Autodesk Fusion 360 part; units mm, degrees
sketch "Esquisse1" plane through (0, 0, 0) normal (0, 0, 1) x (1, 0, 0)
  circle A0 centre (0, 0) radius 6.5
  circle A1 centre (0, 64) radius 6.5
  line L0 (0, 64) -> (0, 0)
  line L1 (0, 64) -> (-6.5, 64)
  line L2 (0, 64) -> (6.5, 64)
  line L3 (0, 0) -> (6.5, 0)
  line L4 (0, 0) -> (-6.5, 0)
  line L5 (-6.5, 64) -> (-6.5, 0)
  line L6 (6.5, 64) -> (6.5, 0)
  line L7 (0, 64) -> (0, 44.5)
  line L8 (-2.75, 47.25) -> (2.75, 47.25)
  circle A2 centre (0, 47.25) radius 2.75
  line L9 (-2.75, 47.25) -> (-6.3285, 62.5166)
  line L10 (2.75, 47.25) -> (6.3285, 62.5166)
  dimension "d1" = 13
  dimension "d2" = 13
  dimension "d3" = 64
  dimension "d4" = 19.5
  dimension "d5" = 5.5
  dimension "d6" = 2.75
  dimension "d7" = 2.75
extrude "Extrusion1" add sketch "Esquisse1" along normal blind 3
extrude "Extrusion2" add sketch "Esquisse1" against normal blind 2 contours A0 L3 L4 | A0 A1 L0 L5 A2 L9 | A0 L0 L4 | A0 L0 L3 | A0 A1 L0 L6 A2 L10
sketch "Esquisse2" plane through (0, 0, 3) normal (0, 0, 1) x (-1, 0, 0)
  line L0 (6.5, -64) -> (6.5, 0)
  arc A0 (6.5, 0) -> (-6.5, 0) centre (0, 0) ccw
  line L1 (-6.5, 0) -> (-6.5, -64)
  arc A1 (-6.5, -64) -> (6.5, -64) centre (0, -64) ccw
  circle A2 centre (0, 0) radius 1.5
  circle A3 centre (0, -64) radius 1.5
  dimension "d12" = 3
  dimension "d13" = 3
extrude "Extrusion3" cut sketch "Esquisse2" against normal blind 5 contours A2 | A3
sketch "Esquisse3" plane through (0, 0, 3) normal (0, 0, 1) x (-1, 0, 0)
  circle A0 centre (0, -64) radius 1.5
  circle A1 centre (0, 0) radius 1.5
  line L0 (6.5, -64) -> (6.5, 0)
  arc A2 (6.5, 0) -> (-6.5, 0) centre (0, 0) ccw
  line L1 (-6.5, 0) -> (-6.5, -64)
  arc A3 (-6.5, -64) -> (6.5, -64) centre (0, -64) ccw
  circle A4 centre (0, -64) radius 1.5
  circle A5 centre (0, -64) radius 3.5
  circle A6 centre (0, 0) radius 1.5
  circle A7 centre (0, 0) radius 3.5
  dimension "d16" = 7
  dimension "d17" = 3
  dimension "d18" = 3
  dimension "d19" = 7
extrude "Extrusion5" add sketch "Esquisse3" along normal blind 2 contours A5 | A7
Source: CAD feature listing. Evaluate the final solid. Frame: model axes, mm. A direction names the side the tool comes from. Coordinates: 2 decimals unless noted, no trailing zeros. Loops run counter-clockwise (first coordinate to the right, second up) from the corner with the lowest first, then second, coordinate; pieces in that order, holes last. Notation, with made-up numbers: M 41.5,-32.5 L 85.5,-32.5 A21 ccw 85.5,-5.5 Z; hole C 29.5,60.5 d5. An arc over 180 degrees is marked long. Use a Markdown table: item, result. Add a question column.
Q1. First-contact query: pin 1 (4 mm diameter, centred on x = 3, z = -0.5, fed in from +Y); pin 2 (1.5 mm diameter, centred on x = 4.5, z = 4, fed in from +Y); pin 3 (4 mm diameter, centred on x = -0.5, y = 57.5, fed in from -Z); pin 4 (1.5 mm diameter, centred on x = -4, y = 56.5, fed in from +Z). Flat tips, straight axial feed; report the tip coordinate or a pass-through.
Q2. Material intervals for L1, parallel to Y at x = 0, z = 1.1; L2, parallel to X at y = 64, z = 1.65; L3, parallel to Y at x = 0, z = 3.2, sorted ascending.
Q3. Section query B-B, the plane z = 2.25. Return loops of the section in (x, y), and give its area (3 significant figures).
Q4. Access query for faces 1 (the cylindrical face through (0.1, -6.5, 0.5)), 2 (the flat face through (0, 58, 0)), 3 (the cylindrical face through (-3.233, -1.341, 3.986)). Directions: +Z, -Z, +X, -X, +Y, -Y. A direction counts if a zero-diameter tool reaches every point of the face in a straight line with its end or side. Return the directions, or none.
Q5. Draft query along X for faces 4 (the cylindrical face through (-0.806, 65.265, 2.465)), 5 (the cylindrical face through (1.5, 0.07, 1.45)), 6 (the flat face through (0, 66, 5)), 7 (the cylindrical face through (-1.88, 66.95, 3.99)). Return one class per face: pulls with the +X half, pulls with the -X half, needs draft (parallel to the pull), parting line crosses it, or undercut.
Q6. Section query A-A, the plane x = 0. Return loops of the section in (y, z), and give its area (3 significant figures).
Q7. Section query D-D, the plane x = 4.75. Return loops of the section in (y, z), and give its area (3 significant figures).
Q8. Section query C-C, the plane z = -1.25. Return loops of the section in (x, y).
Result:
| question | item | result |
|---|---|---|
| 1 | pin 1 | stops at y = 70.41 |
| 1 | pin 2 | passes through |
| 1 | pin 3 | stops at z = 0 |
| 1 | pin 4 | stops at z = 3 |
| 2 | L1 | y = -6.5 to -1.5, 1.5 to 62.5, 65.5 to 70.5 |
| 2 | L2 | x = -6.5 to -1.5, 1.5 to 6.5 |
| 2 | L3 | y = -3.5 to -1.5, 1.5 to 3.5, 60.5 to 62.5, 65.5 to 67.5 |
| 3 | outline | M -6.5,0 A6.5 ccw 6.5,0 L 6.5,64 A6.5 ccw -6.5,64 Z; hole C 0,0 d3; hole C 0,64 d3 |
| 3 | area | 951 mm2 |
| 4 | face 1 | +Z, -Z, -Y |
| 4 | face 2 | -Z, +Y |
| 4 | face 3 | +Z |
| 5 | face 4 | undercut |
| 5 | face 5 | undercut |
| 5 | face 6 | needs draft |
| 5 | face 7 | parting line crosses it |
| 6 | outline | M -6.5,-2 L -1.5,-2 L -1.5,5 L -3.5,5 L -3.5,3 L -6.5,3 Z; M 1.5,-2 L 44.5,-2 L 44.5,0 L 62.5,0 L 62.5,5 L 60.5,5 L 60.5,3 L 3.5,3 L 3.5,5 L 1.5,5 Z; M 65.5,0 L 70.5,0 L 70.5,3 L 67.5,3 L 67.5,5 L 65.5,5 Z |
| 6 | area | 325 mm2 |
| 7 | outline | M -4.44,-2 L 55.78,-2 L 55.78,0 L 68.44,0 L 68.44,3 L -4.44,3 Z |
| 7 | area | 339 mm2 |
| 8 | outline | M -6.5,0 A6.5 ccw 6.5,0 L 6.5,64 A6.5 cw 6.33,62.52 L 2.75,47.25 A2.75 cw -2.75,47.25 L -6.33,62.52 A6.5 cw -6.5,64 Z; hole C 0,0 d3 |
